Part model, mm, in its own coordinate system. A direction names the side the tool comes from. Round coordinates to 2 decimals unless told otherwise and drop trailing zeros. Write each loop counter-clockwise with the first axis right and the second up, starting at its lowest first coordinate (ties: lowest second). Pieces come first, ordered by that corner, then holes. Notation, with made-up numbers: (4, 42.25) -> (37, 42.25) arc R21 cw to (37, 61.25) -> close; hole circle Ø6 at (21, 66). An arc over 180 degrees is marked (long way). Return JSON: item names as keys, results as strings. Group by question number.
Autodesk Inventor part; units mm, degrees
ref_plane "YZ Plane" through (0, 0, 0) normal (1, 0, 0) x (0, 1, 0)
ref_plane "XZ Plane" through (0, 0, 0) normal (0, 1, 0) x (-1, 0, 0)
ref_plane "XY Plane" through (0, 0, 0) normal (0, 0, 1) x (1, 0, 0)
ref_plane "Work Plane1" through (0, 0, 0) normal (0, 0, 1) x (1, 0, 0)
sketch "Sketch1" plane through (0, 0, 0) normal (0, 0, 1) x (1, 0, 0)
  line L0 (475, -625) -> (475, -525) construction
  line L1 (427.5, -425) -> (532.5, -425) construction
  line L2 (175, -525) -> (175, -625) construction
  line L3 (475, -625) -> (175, -625)
  line L4 (175, -625) -> (175, -425)
  line L5 (175, -425) -> (475, -425)
  line L6 (475, -425) -> (475, -625)
  line L7 (460, -610) -> (190, -610)
  line L8 (190, -610) -> (190, -440)
  line L9 (190, -440) -> (460, -440)
  line L10 (460, -440) -> (460, -610)
  line L11 (325, -625) -> (325, -610) construction
  line L12 (475, -525) -> (460, -525) construction
  line L13 (190, -525) -> (175, -525) construction
  line L14 (325, -440) -> (325, -425) construction
  point P0 (0, 0)
  dimension "d0" = 15
extrude "Extrusion1" add sketch "Sketch1" along normal blind 100
sketch "Sketch2" plane through (0, 0, 100) normal (0, 0, 1) x (1, 0, 0)
  line L0 (175, -425) -> (475, -425)
  line L1 (475, -425) -> (475, -625)
  line L2 (475, -625) -> (175, -625)
  line L3 (175, -625) -> (175, -425)
  point P0 (0, 0)
extrude "Extrusion2" add sketch "Sketch2" along normal blind 15
sketch "Sketch3" plane through (175, -625, 0) normal (-1, 0, 0) x (0, 0, 1)
  line L0 (19, 1250) -> (19, 100) construction
  line L1 (0, 100) -> (-19, 100) construction
  line L2 (0, 200) -> (19, 200)
  line L3 (19, 200) -> (19, 100)
  line L4 (19, 100) -> (0, 100)
  line L5 (0, 100) -> (0, 200)
  point P0 (0, 625)
extrude "Extrusion3" cut sketch "Sketch3" against normal up to next
properties part number "Control_Box" material "MDF Medium Density Fiberboard"
Item 1: Wall check: L1, parallel to Y at x = 410, z = 31.5; L2, parallel to X at y = -473, z = 47.5; L3, parallel to Y at x = 313, z = 18.5. Give the ranges that are in metal, low to high.
Item 2: Flat gauge pins, fed straight in: P1, Ø4.5, axis at x = 179.5, z = 5, coming from the +Y side; P2, Ø12, axis at x = 281, y = -554.5, coming from the -Z side. Where does each tip first touch, or does it go through?
Item 3: Two-plate mould, pull along Y, no slides. Class faces 1 (the face through (323, -425, 66)), 2 (the face through (190, -526, 49)), 3 (the face through (323, -524, 100)), 4 (the face through (475, -524, 57)): released by +Y, released by -Y, zero draft, split by the parting line, or undercut.
Item 4: Which spindle directions (+Z, -Z, +X, -X, +Y, -Y) get a long thin tool onto all of the face, cutting with end or side? Do faces 5 (the face through (460, -524, 49)), 6 (the face through (175, -526, 57)), 7 (the face through (182, -525, 10)). Say none if no direction does.
Item 5: Cut at A-A (y = -583). Write the cut outline in (x, z).
Item 6: Cut at C-C (x = 291). Write the cut outline in (y, z).
Item 7: Cut at B-B (z = 32.5). Write the cut outline in (x, y), then the cut area to 3 significant figures.
Checks:
{
 "1": {"L1": "y = -625 to -610, -440 to -425", "L2": "x = 175 to 190, 460 to 475", "L3": "y = -625 to -610"},
 "2": {"P1": "stops at y = -525", "P2": "stops at z = 100"},
 "3": {"face 1": "released by +Y", "face 2": "undercut", "face 3": "undercut", "face 4": "zero draft"},
 "4": {"face 5": "-Z", "face 6": "+Z, -Z, -X, +Y, -Y", "face 7": "-Z, +X, -X, +Y"},
 "5": {"outline": "(175, 0) -> (190, 0) -> (190, 100) -> (460, 100) -> (460, 0) -> (475, 0) -> (475, 115) -> (175, 115) -> close"},
 "6": {"outline": "(-625, 0) -> (-610, 0) -> (-610, 100) -> (-440, 100) -> (-440, 19) -> (-425, 19) -> (-425, 115) -> (-625, 115) -> close"},
 "7": {"outline": "(175, -625) -> (475, -625) -> (475, -425) -> (175, -425) -> close; hole (190, -610) -> (460, -610) -> (460, -440) -> (190, -440) -> close", "area": "14,100 mm2"}
}
